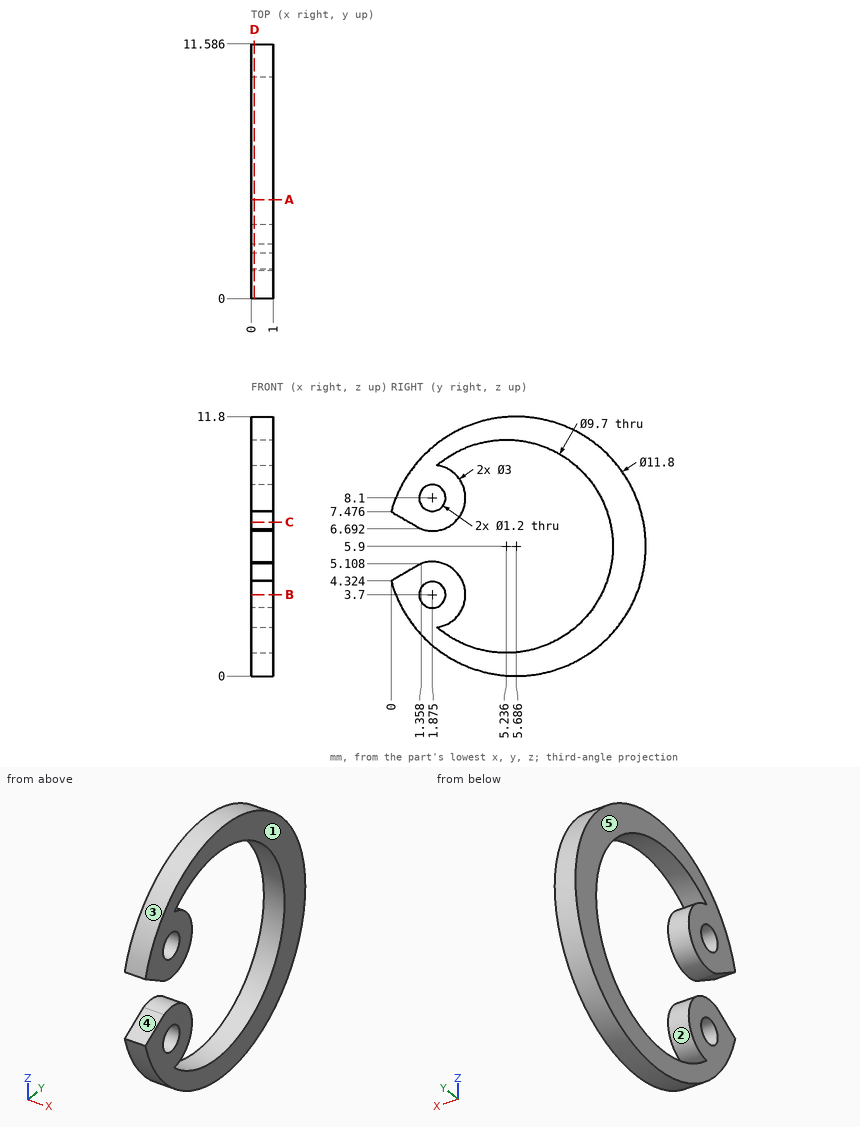
The figure shows three views and two pictorial views of one solid part (mm, origin at its lowest corner). Answer the questions. A direction names the side the tool comes from. Give positions to 0.01 mm unless a question says otherwise; leave off trailing zeros. Order: outer loops, then holes, each group sorted by start corner. A loop starts at its lowest first (then second) coordinate and runs counter-clockwise, first axis right, second up. Notation, with made-up numbers: M 80.5,38.25 L 129.5,38.25 A28 ccw 129.5,76.25 Z; hole C 56,42.5 d7. An arc over 180 degrees is marked long. Return JSON: item names as keys, results as strings.
Q1. Which of the six approach directions +Z, -Z, +X, -X, +Y, -Y give full straight-line access (tool end or side, diameter ignored) to the marked faces 4 and 5?
Answer below:
{"face 4": "+X, -X, -Y", "face 5": "+Z, -Z, -X, +Y, -Y"}
Q2. Find section A-A, the plane y = 4.5. Write down the section's boundary in (x, z).
Answer below:
{"outline": "M 0,0.12 L 1,0.12 L 1,1.11 L 0,1.11 Z; M 0,10.69 L 1,10.69 L 1,11.68 L 0,11.68 Z"}
Q3. Find the intervals of material crossed by line 1 along Z through (x, y) = (0.35, 3.25) (1 decimal); line 2 along Y through (x, z) = (0.45, 8.1) (1 decimal); line 3 along Z through (x, y) = (0.3, 2.75) (1 decimal), in increasing order. Write a range as [from, to].
Answer below:
{"line 1": "z = [0.5, 1.5], [3.1, 4.3], [7.5, 8.7], [10.3, 11.3]", "line 2": "y = [0.2, 1.3], [2.5, 3.4], [9.6, 11.2]", "line 3": "z = [0.8, 1.7], [2.5, 4.9], [6.9, 9.3], [10.1, 11]"}
Q4. Find section C-C, the plane z = 7. Write down the section's boundary in (x, y) (1 decimal).
Answer below:
{"outline": "M 0,0.8 L 1,0.8 L 1,2.9 L 0,2.9 Z; M 0,10 L 1,10 L 1,11.5 L 0,11.5 Z"}
Q5. Find section B-B, the plane z = 3.7. Write down the section's boundary in (x, y) (1 decimal).
Answer below:
{"outline": "M 0,0.2 L 1,0.2 L 1,1.3 L 0,1.3 Z; M 0,2.5 L 1,2.5 L 1,3.4 L 0,3.4 Z; M 0,9.6 L 1,9.6 L 1,11.2 L 0,11.2 Z"}
Q6. The mould has two halves that part along Z. Classify the marked faces 1, 2 and 3: pulls with the +Z half, pulls with the -Z half, needs draft (parallel to the pull), parting line crosses it, or undercut.
Answer below:
{"face 1": "needs draft", "face 2": "undercut", "face 3": "parting line crosses it"}
Q7. Find section D-D, the plane x = 0.15. State how many separate pieces and enclosed holes the cut face has.
Answer below:
{"separate pieces": "1", "enclosed holes": "2"}
